For this review, take the finished solid that the model builds, in its own axes (mm). Face numbers are marked on the shaded views. A direction names the side the tool comes from. Give positions to 0.01 mm unless a question says otherwise; leave off trailing zeros. Loops run counter-clockwise (first coordinate to the right, second up) from the corner with the lowest first, then second, coordinate; pieces in that order, holes last. Notation, with made-up numbers: (47, -13.75) - (52, -13.75) arc R14 cw to (52, -6.75) - close; hole circle Ø3 at (-14.5, 85.5). An arc over 180 degrees is marked (long way). Answer as CSV lines item,"result".
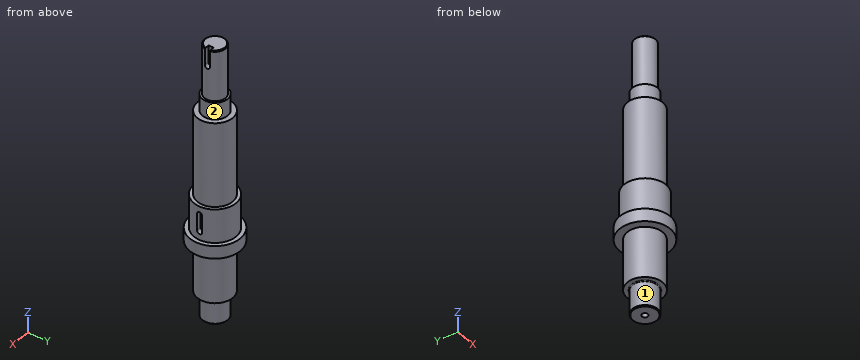
from build123d import *

# Parameters (mm, degrees)
M8X1_0_TAPPED_HOLE1_D     = 7
M8X1_0_TAPPED_HOLE1_DEPTH = 19
M8X1_0_TAPPED_HOLE1_TIP   = 2.103012167
CUT_EXTRUDE3_DEPTH        = 6
CUT_EXTRUDE4_DEPTH        = 6
CHAMFER1_SIZE             = 1
FILLET1_R                 = 1


with BuildPart() as part:
    # Sketch2 → Revolve1 (revolve)
    with BuildSketch(Plane(origin=(0, 0, 0), x_dir=(0, 0, -1), z_dir=(1, 0, 0))):
        Polygon((-225, 12.5), (-225, 0), (100, 0), (100, 15), (70, 15), (70, 21), (10, 21), (10, 30), (-5, 30), (-5, 25), (-45, 25), (-45, 21), (-145, 21), (-145, 15), (-165, 15), (-165, 12.5), align=None)
    revolve(axis=Axis((0, 0, 225), (0, 0, -1)))

    # M8x1.0 Tapped Hole1
    with Locations(Plane(origin=(0, 0, -100), x_dir=(0, -1, 0), z_dir=(0, 0, -1))):
        with Locations((0, 0)):
            Hole(M8X1_0_TAPPED_HOLE1_D / 2, depth=M8X1_0_TAPPED_HOLE1_DEPTH)
            with Locations((0, 0, -(M8X1_0_TAPPED_HOLE1_DEPTH + M8X1_0_TAPPED_HOLE1_TIP / 2))):  # 118° drill point
                Cone(0, M8X1_0_TAPPED_HOLE1_D / 2, M8X1_0_TAPPED_HOLE1_TIP, mode=Mode.SUBTRACT)

    # Sketch4 → Cut-Extrude3 (cut)
    with BuildSketch(Plane(origin=(12.5, 0, 0), x_dir=(0, 0, -1), z_dir=(1, 0, 0))):
        with BuildLine():
            Line((-205, 3), (-225, 3))
            Line((-225, 3), (-225, -3))
            Line((-225, -3), (-205, -3))
            ThreePointArc((-205, -3), (-202, 0), (-205, 3))
        make_face()
    extrude(amount=-CUT_EXTRUDE3_DEPTH, mode=Mode.SUBTRACT)

    # Sketch5 → Cut-Extrude4 (cut)
    with BuildSketch(Plane(origin=(25, 0, 0), x_dir=(0, 0, -1), z_dir=(1, 0, 0))):
        with BuildLine():
            Line((-35, 3), (-15, 3))
            ThreePointArc((-15, 3), (-12, 0), (-15, -3))
            Line((-15, -3), (-35, -3))
            ThreePointArc((-35, -3), (-38, 0), (-35, 3))
        make_face()
    extrude(amount=-CUT_EXTRUDE4_DEPTH, mode=Mode.SUBTRACT)

    # Chamfer1
    chamfer1_edges = [part.edges().sort_by_distance(p)[0] for p in [
        (0, -15, -100),
        (-9.842509843, -7.705517504, 225),
    ]]
    chamfer(chamfer1_edges, length=CHAMFER1_SIZE)

    # Fillet1
    fillet1_edges = [part.edges().sort_by_distance(p)[0] for p in [
        (0, -15, -70),
    ]]
    fillet(fillet1_edges, radius=FILLET1_R)


solid = part.part
1) Consider section A-A on z = 67. Write out the cut boundary in (x, y), and give its area (3 significant figures).
From the geometry:
outline,"circle Ø42 at (0, 0)"
area,"1,390 mm^2"
2) Consider section B-B on z = 184.5. Write out the cut boundary in (x, y), and give its area (3 significant figures).
From the geometry:
outline,"circle Ø25 at (0, 0)"
area,"491 mm^2"
3) Machinability: for the marked faces 1 and 2, which of the approach directions +Z, -Z, +X, -X, +Y, -Y give a long, thin tool a straight path to every point of the face, cutting with its end or side? Answer none if there is none.
From the geometry:
face 1,"-Z"
face 2,"+Z"
4) Wall thickness on line 1 (X direction, y = 0, z = -88.75); line 2 (Z direction, x = 15, y = -17.5); line 3 (Z direction, x = 17, y = -2): over which ranges is each line inside the solid? List them lowest first. Write a range as from..to.
From the geometry:
line 1,"x = -15..-3.5, 3.5..15"
line 2,"z = -10..45"
line 3,"z = -70..145"
5) Insertion check: P1, Ø4, axis at x = 18.5, y = 0.5, coming from the +Z side; P2, Ø6, axis at x = -17, y = -8.5, coming from the -Z side; P3, Ø1.5, axis at y = -19.5, z = 88, coming from the -X side. Each pin has a flat end and moves straight along its axis. Give the tip position at first contact, or say it passes through.
From the geometry:
P1,"stops at z = 145"
P2,"stops at z = -70"
P3,"stops at x = -9.46"
